Check sheet for the modelled part. Datum: model origin and axes. Units: mm. Give positions to 0.01 mm unless a question says otherwise; leave off trailing zeros. Loops run counter-clockwise (first coordinate to the right, second up) from the corner with the lowest first, then second, coordinate; pieces in that order, holes last.
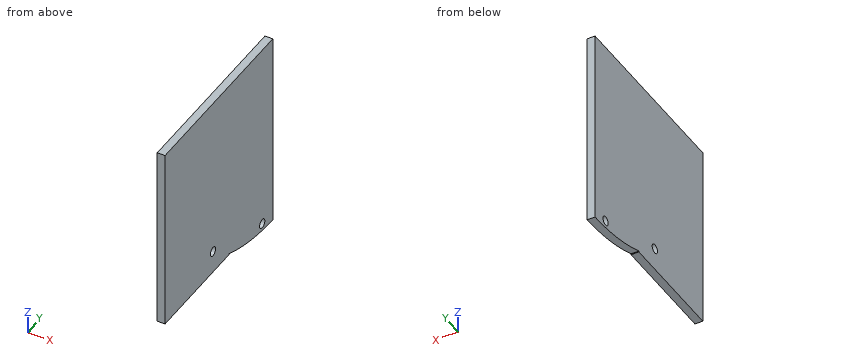
```python
from build123d import *

# Parameters (mm, degrees)
SKETCH1_R           = 3.175
BOSS_EXTRUDE2_DEPTH = 5.4102


with BuildPart() as part:
    # Sketch1 → Boss-Extrude2 (new body)
    with BuildSketch(Plane(origin=(0, 0, 0), x_dir=(0, 0, -1), z_dir=(1, 0, 0))):
        with BuildLine():
            Line((139.192, 0), (0, 0))
            Line((0, 0), (0, -129.54))
            Line((0, -129.54), (129.54, -129.54))
            Line((129.54, -129.54), (129.54, -52.681426173))
            Line((129.54, -52.681426173), (128.837417703, -52.681426173))
            ThreePointArc((128.837417703, -52.681426173), (136.578824693, -26.844692391), (139.192, 0))
        make_face()
        with Locations((113.804702463, -71.909902638)):
            Circle(SKETCH1_R, mode=Mode.SUBTRACT)
        with Locations((133.35, -12.7)):
            Circle(SKETCH1_R, mode=Mode.SUBTRACT)
    extrude(amount=BOSS_EXTRUDE2_DEPTH)


solid = part.part
```
(1) Section check C-C on z = -133.35. Record the boundary of the cut face in (x, y) (3 decimals).
(2) Section check B-B on x = 2.9. Record the boundary of the cut face in (y, z) (3 decimals), plus the area to 3 significant figures.
(3) Gauge pin test, flat end, axial feed: pin 1 Ø2.5 at (x, y) = (3.5, -97) entering from -Z. Record the tip position at first contact, or that the pin passes through.
(4) Section check D-D on y = -65.5. Record the boundary of the cut face in (x, z).
(5) Section check A-A on y = -12.7. Record the boundary of the cut face in (x, z) (3 decimals), plus the area to 3 significant figures.
(6) Material ranges on line 1 (Z direction, x = 3.9, y = -122); line 2 (Z direction, x = 1.8, y = -73.5); line 3 (Z direction, x = 2.45, y = -14), recorded low to high.
Computed values:
1. outline: (0, -39.902) - (5.41, -39.902) - (5.41, -15.875) - (0, -15.875) - close; (0, -9.525) - (5.41, -9.525) - (5.41, 0) - (0, 0) - close
2. outline: (-129.54, -129.54) - (-52.681, -129.54) - (-52.681, -128.837) arc R139.192 ccw to (0, -139.192) - (0, 0) - (-129.54, 0) - close; hole circle Ø6.35 at (-71.91, -113.805); hole circle Ø6.35 at (-12.7, -133.35)
2. area: 17,000 mm2
3. pin 1: stops at z = -129.54
4. outline: (0, -129.54) - (5.41, -129.54) - (5.41, 0) - (0, 0) - close
5. outline: (0, -138.611) - (5.41, -138.611) - (5.41, -136.525) - (0, -136.525) - close; (0, -130.175) - (5.41, -130.175) - (5.41, 0) - (0, 0) - close
5. area: 716 mm2
6. line 1: z = -129.54 to 0
6. line 2: z = -129.54 to -116.55, -111.06 to 0
6. line 3: z = -138.49 to -136.25, -130.45 to 0
